Here's the drawing with two shaded views (mm, measured from the low corner). I have some questions. Coordinates: 2 decimals unless noted, no trailing zeros. Write each loop counter-clockwise with the first axis right and the second up, starting at its lowest first coordinate (ties: lowest second). Pieces come first, ordered by that corner, then holes. Notation, with made-up numbers: (53, 76) - (79, 76) arc R17 cw to (79, 86) - close; hole circle Ø6 at (42, 50.25). An arc over 180 degrees is marked (long way). Answer in a Markdown table with one row per item. Add a question column.
Item 1: I'm going to push flat-ended pins straight in: pin 1 (2.5 mm diameter, centred on y = 98.5, z = 4.5, fed in from +X); pin 2 (1 mm diameter, centred on y = 110.5, z = 5, fed in from -X); pin 3 (1.5 mm diameter, centred on x = 43, y = 73, fed in from -Z); pin 4 (1.6 mm diameter, centred on x = 145.5, z = 5.5, fed in from +Y). Where does each tip first touch, or does it pass through?
Item 2: Imagine slicing it at D-D (x = 73.5). Please give me the cut outline in (y, z) (3 decimals), plus the area to 3 significant figures.
Item 3: If I drill on probe 1 along Y at (x, z) = (101.6, 3); probe 2 along Y at (x, z) = (101.6, 3.75); probe 3 along Y at (x, z) = (137, 5), over which ranges is the centre line in solid material (lowest first)? Write a range as from..to.
Item 4: Imagine slicing it at C-C (z = 4.5). Please give me the cut outline in (x, y) (1 decimal).
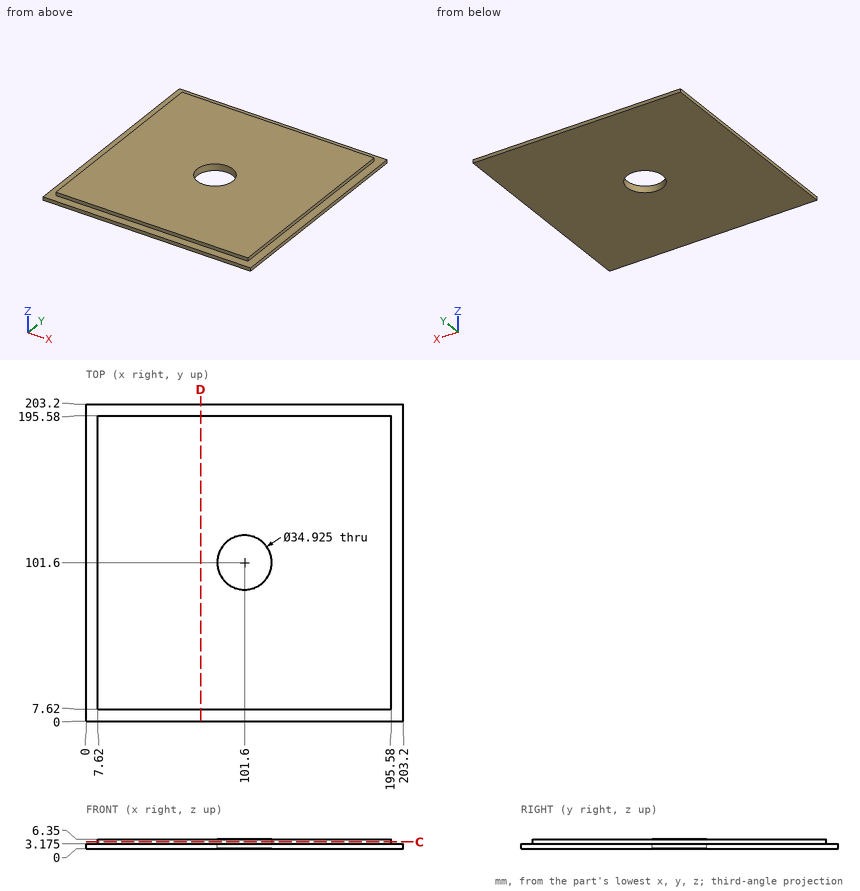
Here are the results:
| question | item | result |
|---|---|---|
| 1 | pin 1 | stops at x = 195.58 |
| 1 | pin 2 | stops at x = 7.62 |
| 1 | pin 3 | stops at z = 0 |
| 1 | pin 4 | stops at y = 195.58 |
| 2 | outline | (0, 0) - (203.2, 0) - (203.2, 3.175) - (195.58, 3.175) - (195.58, 6.35) - (7.62, 6.35) - (7.62, 3.175) - (0, 3.175) - close |
| 2 | area | 1,240 mm2 |
| 3 | probe 1 | y = 0..84.14, 119.06..203.2 |
| 3 | probe 2 | y = 7.62..84.14, 119.06..195.58 |
| 3 | probe 3 | y = 7.62..195.58 |
| 4 | outline | (7.6, 7.6) - (195.6, 7.6) - (195.6, 195.6) - (7.6, 195.6) - close; hole circle Ø34.9 at (101.6, 101.6) |
